Autodesk Inventor part; units mm, degrees
ref_plane "YZ Plane" through (0, 0, 0) normal (1, 0, 0) x (0, 1, 0)
ref_plane "XZ Plane" through (0, 0, 0) normal (0, 1, 0) x (-1, 0, 0)
ref_plane "XY Plane" through (0, 0, 0) normal (0, 0, 1) x (1, 0, 0)
sketch "Sketch1" plane through (0, 0, 0) normal (1, 0, 0) x (0, 1, 0)
  line L0 (25, 25) -> (-25, 25)
  line L1 (-25, 25) -> (-25, -25)
  line L2 (-25, -25) -> (25, -25)
  line L3 (25, -25) -> (25, 25)
  line L4 (25, 25) -> (-25, -25) construction
  line L5 (-25, 25) -> (25, -25) construction
  circle A0 centre (0, 0) radius 4
  dimension "d0" = 50
  dimension "d1" = 50
  dimension "d11" = 8
extrude "Extrusion1" add sketch "Sketch1" along normal blind 2
sketch "Sketch2" plane through (0, -25, 25) normal (0, 0, 1) x (1, 0, 0)
  line L0 (2, 0) -> (52, 0)
  line L1 (52, 0) -> (52, 10)
  line L2 (2, 0) -> (2, 50)
  line L3 (2, 50) -> (12, 50)
  line L4 (12, 50) -> (52, 10)
  point P0 (0, 25)
  dimension "d4" = 50
  dimension "d5" = 10
  dimension "d6" = 10
extrude "Extrusion2" add sketch "Sketch2" against normal blind 2
sketch "Sketch3" plane through (0, -25, -25) normal (0, 0, -1) x (-1, 0, 0)
  line L0 (-52, 0) -> (-2, 0)
  line L1 (-2, 50) -> (-2, 0)
  line L2 (-2, 50) -> (-12, 50)
  line L3 (-12, 50) -> (-52, 10)
  line L4 (-52, 10) -> (-52, 0)
  point P0 (0, 25)
extrude "Extrusion3" add sketch "Sketch3" against normal blind 2
properties part number "Tensioner_fix"
Here's how the part is built. I have some questions about the finished solid (model axes, mm). A direction names the side the tool comes from. Give positions to 0.01 mm unless a question says otherwise; leave off trailing zeros. Loops run counter-clockwise (first coordinate to the right, second up) from the corner with the lowest first, then second, coordinate; pieces in that order, holes last. Notation, with made-up numbers: M 24.25,-36.5 L 67.25,-36.5 A19 ccw 67.25,-1.5 Z; hole C 33,-31 d8. An arc over 180 degrees is marked long. Put each result on its own line as item: value. Start each with the question number.
(1) I want a section at B-B on y = 0. Please give me the cut outline in (x, z), then the cut area to 3 significant figures.
(2) If we mould it in two halves opening along Z, with no side actions, what happens to faces 3 (the flat face through (21, -5, 23)), 4 (the flat face through (52, -20, -24)), 5 (the cylindrical face through (0.986, -0.867, 3.905)), 6 (the flat face through (21, -5, -25))? For each: +Z half, -Z half, draft (parallel to the pull), parting line (faces both ways), or undercut.
(3) For faces 1 (the flat face through (2, 0, 5)), 2 (the flat face through (32, 5, -24)), which set-ups out of +Z, -Z, +X, -X, +Y, -Y let a thin tool reach every point of the face, with its end or its side?
(4) Will this pin go through, and if not, where does the flat tip stop? pin 1 Ø1.5 at (y, z) = (-2, -3) entering from +X.
(5) I need wall thicknesses on line 1 along Z through (x, y) = (20, -5); line 2 along Z through (x, y) = (1, 0); line 3 along X through (y, z) = (10.5, 8.5). Which ranges of each line are inside material? Lowest first, please. Write a range as [from, to].
(6) I want a section at C-C on z = 0. Please give me the cut outline in (x, y), then the cut area to 3 significant figures.
(7) I want a section at D-D on y = 6.5. Please give me the cut outline in (x, z), then the cut area to 3 significant figures.
(8) I want a section at A-A on x = 42. Please give me the cut outline in (y, z).
Answer block:
1. outline: M 0,-25 L 37,-25 L 37,-23 L 2,-23 L 2,-4 L 0,-4 Z; M 0,4 L 2,4 L 2,23 L 37,23 L 37,25 L 0,25 Z
1. area: 224 mm^2
2. face 3: undercut
2. face 4: draft
2. face 5: undercut
2. face 6: -Z half
3. face 1: +X, +Y, -Y
3. face 2: +Z, -Z, +X, +Y
4. pin 1: x = 2
5. line 1: [-25, -23], [23, 25]
5. line 2: [-25, -4], [4, 25]
5. line 3: [0, 2]
6. outline: M 0,-25 L 2,-25 L 2,-4 L 0,-4 Z; M 0,4 L 2,4 L 2,25 L 0,25 Z
6. area: 84.0 mm^2
7. outline: M 0,-25 L 30.5,-25 L 30.5,-23 L 2,-23 L 2,23 L 30.5,23 L 30.5,25 L 0,25 Z
7. area: 214 mm^2
8. outline: M -25,-25 L -5,-25 L -5,-23 L -25,-23 Z; M -25,23 L -5,23 L -5,25 L -25,25 Z
